```python
from build123d import *

# Parameters (mm, degrees)
F0_W     = 30
F0_H     = 21
F0_R     = 4
F1_DEPTH = 35
F2_R     = 7
F3_DEPTH = 5.5
F4_R     = 7
F5_DEPTH = 5.5
F6_R     = 1.75
F7_DEPTH = 21


with BuildPart() as f1:
    # F0 (on Top) → F1 (new body)
    with BuildSketch(Plane.XY):
        Rectangle(F0_W, F0_H)
        Circle(F0_R, mode=Mode.SUBTRACT)
    extrude(amount=F1_DEPTH)

    # F2 (on face) → F3 (cut)
    with BuildSketch(Plane.XY.offset(35)):
        Circle(F2_R)
    extrude(amount=-F3_DEPTH, mode=Mode.SUBTRACT)

    # F4 (on face) → F5 (cut)
    with BuildSketch(Plane(origin=(0, 0, 0), x_dir=(1, 0, 0), z_dir=(0, 0, -1))):
        Circle(F4_R)
    extrude(amount=-F5_DEPTH, mode=Mode.SUBTRACT)

    # F6 (on face) → F7 (cut, through all)
    with BuildSketch(Plane.XZ.offset(10.5)):
        with Locations((8.89, 5.562)):
            Circle(F6_R)
        with Locations((-8.89, 5.562)):
            Circle(F6_R)
        with Locations((8.89, 29.438)):
            Circle(F6_R)
        with Locations((-8.89, 29.438)):
            Circle(F6_R)
    extrude(amount=-F7_DEPTH, mode=Mode.SUBTRACT)


solid = f1.part
```
The listing builds one solid part. Answer for the finished solid, in the listing's coordinates (mm). A direction names the side the tool comes from. Give positions to 0.01 mm unless a question says otherwise; leave off trailing zeros. Order: outer loops, then holes, each group sorted by start corner. A loop starts at its lowest first (then second) coordinate and runs counter-clockwise, first axis right, second up. Notation, with made-up numbers: (-11.75, 74) -> (24.25, 74) arc R11 ccw to (24.25, 81) -> close; hole circle Ø10 at (-15.75, -8). An arc over 180 degrees is marked (long way). One line per item, written item: value.
1) A flat-ended cylindrical pin translates along its axis: P1, Ø8.5, axis at x = 0, y = 0, coming from the +Z side. Find the tip coordinate at first contact, or state that the pin passes through.
Reported:
P1: stops at z = 29.5
2) Find the intervals of material crossed by line 1 (Z direction, x = 8.89, y = 6); line 2 (Y direction, x = 0, z = 11.75); line 3 (Z direction, x = -8, y = -8), in increasing order.
Reported:
line 1: z = 0 to 3.81, 7.31 to 27.69, 31.19 to 35
line 2: y = -10.5 to -4, 4 to 10.5
line 3: z = 0 to 4.06, 7.07 to 27.93, 30.94 to 35
3) Find section A-A, the plane y = -3. Determine the outline of the cut face in (x, z).
Reported:
outline: (-15, 0) -> (-6.32, 0) -> (-6.32, 5.5) -> (-2.65, 5.5) -> (-2.65, 29.5) -> (-6.32, 29.5) -> (-6.32, 35) -> (-15, 35) -> close; (2.65, 5.5) -> (6.32, 5.5) -> (6.32, 0) -> (15, 0) -> (15, 35) -> (6.32, 35) -> (6.32, 29.5) -> (2.65, 29.5) -> close; hole circle Ø3.5 at (-8.89, 5.56); hole circle Ø3.5 at (-8.89, 29.44); hole circle Ø3.5 at (8.89, 5.56); hole circle Ø3.5 at (8.89, 29.44)
4) A tool of negligible diameter and unlimited length cuts with its end or side. For faces 4 (the flat face through (3, -3, 29.5)), 5 (the cylindrical face through (-7.22, -0.15, 6.09)), 6 (the cylindrical face through (6.466, 2.681, 2.712)), from which of +Z, -Z, +X, -X, +Y, -Y can it reach the whole face along a straight path? Write none if from no direction.
Reported:
face 4: +Z
face 5: +Y, -Y
face 6: -Z
5) Find section C-C, the plane z = 6. Determine the outline of the cut face in (x, y).
Reported:
outline: (-15, -10.5) -> (-10.58, -10.5) -> (-10.58, 10.5) -> (-15, 10.5) -> close; (-7.2, -10.5) -> (7.2, -10.5) -> (7.2, 10.5) -> (-7.2, 10.5) -> close; (10.58, -10.5) -> (15, -10.5) -> (15, 10.5) -> (10.58, 10.5) -> close; hole circle Ø8 at (0, 0)
6) Determine the mould class of faces 1 (the flat face through (-15, 0, 17)), 2 (the flat face through (3, 3, 5.5)), 3 (the flat face through (0, 10.5, 17)) for opening direction X: pulls with the +X half, pulls with the -X half, needs draft (parallel to the pull), parting line crosses it, or undercut.
Reported:
face 1: pulls with the -X half
face 2: undercut
face 3: needs draft
7) Find section D-D, the plane x = 8.89. Determine the outline of the cut face in (y, z), plus the area to 3 significant figures.
Reported:
outline: (-10.5, 0) -> (10.5, 0) -> (10.5, 3.81) -> (-10.5, 3.81) -> close; (-10.5, 7.31) -> (10.5, 7.31) -> (10.5, 27.69) -> (-10.5, 27.69) -> close; (-10.5, 31.19) -> (10.5, 31.19) -> (10.5, 35) -> (-10.5, 35) -> close
area: 588 mm^2
8) Find section B-B, the plane x = 0. Determine the outline of the cut face in (y, z).
Reported:
outline: (-10.5, 0) -> (-7, 0) -> (-7, 5.5) -> (-4, 5.5) -> (-4, 29.5) -> (-7, 29.5) -> (-7, 35) -> (-10.5, 35) -> close; (4, 5.5) -> (7, 5.5) -> (7, 0) -> (10.5, 0) -> (10.5, 35) -> (7, 35) -> (7, 29.5) -> (4, 29.5) -> close
